Check sheet for the modelled part. Datum: model origin and axes. Units: mm. Face numbers are marked on the shaded views. A direction names the side the tool comes from. Round coordinates to 2 decimals unless told otherwise and drop trailing zeros. Write each loop counter-clockwise with the first axis right and the second up, starting at its lowest first coordinate (ties: lowest second). Pieces come first, ordered by that corner, then holes. Notation, with made-up numbers: (1, 72.25) -> (54, 72.25) arc R21 ccw to (54, 76.25) -> close; hole circle Ø6 at (54.5, 43.5). An arc over 180 degrees is marked (long way). One line per item, written item: value.
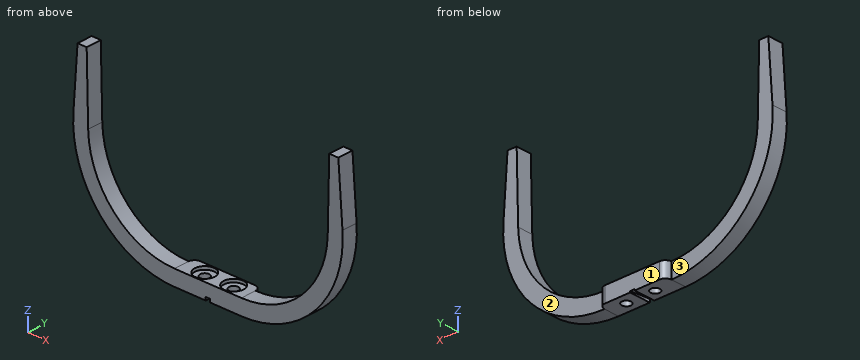
Autodesk Inventor part; units mm, degrees
ref_plane "YZ Plane" through (0, 0, 0) normal (1, 0, 0) x (0, 1, 0)
ref_plane "XZ Plane" through (0, 0, 0) normal (0, 1, 0) x (-1, 0, 0)
ref_plane "XY Plane" through (0, 0, 0) normal (0, 0, 1) x (1, 0, 0)
ref_plane "Work Plane1" through (0, 0, 0) normal (0, 0, 1) x (1, 0, 0)
sketch "Sketch1" plane through (0, 0, 0) normal (0, 0, 1) x (1, 0, 0)
  circle A0 centre (10.2273, -23.9687) radius 0.75
  circle A1 centre (0.7, 24) radius 0.75
  circle A2 centre (10.2, 24) radius 0.75
  circle A3 centre (0.7, -24) radius 0.75
  arc A4 (-14, 7) -> (-16, 5) centre (-14, 5) ccw
  line L0 (-16, -15) -> (-16, 5)
  arc A5 (-16, -15) -> (-14, -17) centre (-14, -15) ccw
  line L1 (-8, -17) -> (-14, -17)
  arc A6 (-6, -19) -> (-8, -17) centre (-8, -19) ccw
  line L2 (-6, -25.5) -> (-6, -19)
  arc A7 (-6, -25.5) -> (-4, -27.5) centre (-4, -25.5) ccw
  line L3 (14, -27.5) -> (-4, -27.5)
  arc A8 (14, -27.5) -> (16, -25.5) centre (14, -25.5) ccw
  line L4 (16, -20.5) -> (16, -25.5)
  line L5 (-4, -20.5) -> (16, -20.5)
  line L6 (-4, -15) -> (-4, -20.5)
  line L7 (-14, -15) -> (-4, -15)
  line L8 (-14, 5) -> (-14, -15)
  line L9 (-4, 5) -> (-14, 5)
  line L10 (-4, 20.5) -> (-4, 5)
  line L11 (16, 20.5) -> (-4, 20.5)
  line L12 (16, 25.5) -> (16, 20.5)
  arc A9 (16, 25.5) -> (14, 27.5) centre (14, 25.5) ccw
  line L13 (-4, 27.5) -> (14, 27.5)
  arc A10 (-4, 27.5) -> (-6, 25.5) centre (-4, 25.5) ccw
  line L14 (-6, 9) -> (-6, 25.5)
  arc A11 (-8, 7) -> (-6, 9) centre (-8, 9) ccw
  line L15 (-14, 7) -> (-8, 7)
  line L16 (-4, 20.5) -> (-6, 20.5)
  point P0 (0, 0)
extrude "Extrusion1" add sketch "Sketch1" along normal blind 5 contours L14 A10 L13 A9 L12 L11 L16
sketch "Sketch2" plane through (0, 0, 5) normal (0, 0, 1) x (1, 0, 0)
  circle A0 centre (0.7, 24) radius 0.75
  circle A1 centre (10.2, 24) radius 0.75
  point P0 (0, 0)
hole "Hole1" at (0.7, 24, 5) at (10.2, 24, 5) direction (0, 0, -1) diameter 3 end through all counterbore diameter 6.5 counterbore depth 1
sketch "Sketch4" plane through (-6, 20.5, 0) normal (0, -1, 0) x (1, 0, 0)
  line L0 (0, 0) -> (22, 0)
  line L1 (11.75, -1) -> (10.25, -1) construction
  line L2 (10.25, -1) -> (10.25, 1) construction
  line L3 (10.25, 1) -> (11.75, 1) construction
  line L4 (11.75, 1) -> (11.75, -1) construction
  line L5 (11.75, -1) -> (10.25, 1) construction
  line L6 (10.25, -1) -> (11.75, 1) construction
  line L7 (10.25, 1) -> (11.75, 1)
  line L8 (11.75, 1) -> (11.75, 0)
  line L9 (11.75, 0) -> (10.25, 0)
  line L10 (10.25, 0) -> (10.25, 1)
  point P0 (6, 0)
  point P1 (11, 0)
  dimension "d9" = 1.5
  dimension "d10" = 2
extrude "Extrusion2" cut sketch "Sketch4" against normal through all
draft "FaceDraft1" angle 5 pull direction (0, -1, 0) faces at (5.25, 22.8333, 1) fixed edges at (5, 20.5, 1)
sketch "Sketch5" plane through (-6, 20.5, 5) normal (0, -1, 0) x (1, 0, 0)
  arc A0 (-33.2285, 30.645) -> (0, -5) centre (0, 28.3104) ccw
  line L0 (2, 0) -> (0, 0)
  arc A1 (-28.3785, 27.7601) -> (0, 0) centre (0, 28.3854) ccw
  line L1 (-33.2285, 30.645) -> (-31.8686, 50)
  line L2 (-31.8686, 50) -> (-28.8686, 50)
  line L3 (-28.8686, 50) -> (-28.3785, 27.7601)
  line L4 (0, 0) -> (22, 0)
  line L5 (0, -5) -> (10.25, -5)
  line L6 (0, -5) -> (0, 0)
  line L7 (0, -5) -> (0, 0)
  dimension "d15" = 50
  dimension "d16" = 3
ref_plane "Work Plane2" through (5, 20.5, 0) normal (1, 0, 0) x (0, 0, -1)
extrude "Extrusion3" add sketch "Sketch5" against normal blind 5
mirror "Mirror1" about plane through (5, 20.5, 0) normal (1, 0, 0) of "Extrusion3"
properties part number "leg"
Item 1: Sectioned sample at C-C (y = 24). State how many separate pieces and enclosed holes the cut face has, then the cut area to 3 significant figures.
Result set:
separate pieces: 3
enclosed holes: 0
area: 727 mm^2
Item 2: Sectioned sample at B-B (z = 28.5). Enter the section's corners in (x, y), then the cut area to 3 significant figures.
Result set:
outline: (-38.96, 20.5) -> (-33.96, 20.5) -> (-33.96, 25.5) -> (-38.96, 25.5) -> close; (43.96, 20.5) -> (48.96, 20.5) -> (48.96, 25.5) -> (43.96, 25.5) -> close
area: 50.0 mm^2
Item 3: Sectioned sample at A-A (x = 10.2). Enter the section's corners in (y, z).
Result set:
outline: (20.5, 0) -> (22.5, 0) -> (22.5, 4) -> (20.75, 4) -> (20.75, 5) -> (20.5, 5) -> close; (25.5, 0) -> (27.5, 0) -> (27.5, 5) -> (27.25, 5) -> (27.25, 4) -> (25.5, 4) -> close
Item 4: Depth check by flat-ended pin: pin 1 (1.5 mm diameter, centred on x = -9, y = 25.5, fed in from +Z); pin 2 (16.5 mm diameter, centred on x = -26.5, z = 34.5, fed in from +Y); pin 3 (1 mm diameter, centred on y = 23.5, z = 45, fed in from +X); pin 4 (1 mm diameter, centred on x = -28, z = 17.5, fed in from -Y). Enter the tip coordinate at first touch or a pass-through.
Result set:
pin 1: z = 5.25
pin 2: y = 25.5
pin 3: x = 48.61
pin 4: through
Item 5: Tool access check on the marked faces 1, 2 and 3. Record the directions out of +Z, -Z, +X, -X, +Y, -Y that give a thin tool (end or side, any length) a straight path to the whole face; none if there is none.
Result set:
face 1: +Z, -Z, +X, -X, +Y
face 2: +Z, -Z, +X, +Y
face 3: +Z, -Z, -X, +Y
Item 6: Sectioned sample at D-D (z = 36.5). Enter the section's corners in (x, y), then the cut area to 3 significant figures.
Result set:
outline: (-39.17, 20.5) -> (-34.46, 20.5) -> (-34.46, 25.5) -> (-39.17, 25.5) -> close; (44.46, 20.5) -> (49.17, 20.5) -> (49.17, 25.5) -> (44.46, 25.5) -> close
area: 47.1 mm^2
Item 7: Material ranges on line 1 along Y through (x, z) = (0.7, 4.7); line 2 along Y through (x, z) = (10, 1); line 3 along Y through (x, z) = (24.5, 5), recorded low to high.
Result set:
line 1: 20.5 to 20.75, 27.25 to 27.5
line 2: 20.5 to 22.51, 25.49 to 27.5
line 3: 20.5 to 25.5
